from build123d import *

# Parameters (mm, degrees)
SKETCH1_W           = 25.4
SKETCH1_H           = 88.9
BOSS_EXTRUDE1_DEPTH = 30.226
SKETCH2_R           = 3.175
CUT_EXTRUDE1_DEPTH  = 12.7
SKETCH3_R           = 8.763
CUT_EXTRUDE2_DEPTH  = 3.556
CUT_EXTRUDE3_START  = -21.844
SKETCH4_R           = 10.795
CUT_EXTRUDE3_DEPTH  = 21.844
SKETCH5_W           = 54.61
SKETCH5_H           = 30.226
BOSS_EXTRUDE2_DEPTH = 3.175
SKETCH6_R           = 1.5875
CUT_EXTRUDE4_DEPTH  = 3.175
BOSS_EXTRUDE3_START = 2.54
SKETCH8_R           = 10.795
SKETCH8_R_2         = 6.35
BOSS_EXTRUDE3_DEPTH = 2.54
BOSS_EXTRUDE4_START = 19.304
SKETCH9_R           = 10.795
BOSS_EXTRUDE4_DEPTH = 19.304
SKETCH10_R          = 8.763
BOSS_EXTRUDE5_DEPTH = 10.16
SKETCH12_R          = 4.445
CUT_EXTRUDE5_DEPTH  = 12.7


with BuildPart() as part:
    # Sketch1 → Boss-Extrude1 (new body)
    with BuildSketch(Plane.XY):
        Rectangle(SKETCH1_W, SKETCH1_H)
    extrude(amount=BOSS_EXTRUDE1_DEPTH)

    # Sketch2 → Cut-Extrude1 (cut)
    with BuildSketch(Plane(origin=(12.7, 0, 0), x_dir=(0, 0, -1), z_dir=(1, 0, 0))):
        with Locations((-15.113, 38.1)):
            Circle(SKETCH2_R)
        with Locations((-15.113, -38.1)):
            Circle(SKETCH2_R)
    extrude(amount=-CUT_EXTRUDE1_DEPTH, mode=Mode.SUBTRACT)

    # Sketch3 → Cut-Extrude2 (cut)
    with BuildSketch(Plane(origin=(12.7, 0, 0), x_dir=(0, 0, -1), z_dir=(1, 0, 0))):
        with Locations((-15.113, 0)):
            Circle(SKETCH3_R)
    extrude(amount=-CUT_EXTRUDE2_DEPTH, mode=Mode.SUBTRACT)

    # Sketch4 → Cut-Extrude3 (cut)
    with BuildSketch(Plane(origin=(9.144, 0, 0), x_dir=(0, 0, -1), z_dir=(1, 0, 0)).offset(CUT_EXTRUDE3_START)):
        with Locations((-15.113, 0)):
            Circle(SKETCH4_R)
    extrude(amount=CUT_EXTRUDE3_DEPTH, mode=Mode.SUBTRACT)

    # Sketch5 → Boss-Extrude2 (add)
    with BuildSketch(Plane.XZ.offset(44.45)):
        with Locations((0, 15.113)):
            Rectangle(SKETCH5_W, SKETCH5_H)
    extrude(amount=BOSS_EXTRUDE2_DEPTH)

    # Sketch6 → Cut-Extrude4 (cut)
    with BuildSketch(Plane.XZ.offset(47.625)):
        with Locations(Location((-23.495, 25.908, 0), (0, 0, 270))):
            Circle(SKETCH6_R)
        with Locations(Location((-23.495, 4.318, 0), (0, 0, 270))):
            Circle(SKETCH6_R)
        with Locations(Location((23.495, 4.318, 0), (0, 0, 270))):
            Circle(SKETCH6_R)
        with Locations(Location((23.495, 25.908, 0), (0, 0, 270))):
            Circle(SKETCH6_R)
    extrude(amount=-CUT_EXTRUDE4_DEPTH, mode=Mode.SUBTRACT)

    # Sketch8 → Boss-Extrude3 (add)
    with BuildSketch(Plane.ZY.offset(-9.144).offset(BOSS_EXTRUDE3_START)):
        with Locations(Location((15.113, 0, 0), (0, 0, 180))):
            Circle(SKETCH8_R)
        with Locations((15.113, 0)):
            Circle(SKETCH8_R_2, mode=Mode.SUBTRACT)
    extrude(amount=-BOSS_EXTRUDE3_DEPTH)

    # Sketch9 → Boss-Extrude4 (add)
    with BuildSketch(Plane.ZY.offset(-6.604).offset(BOSS_EXTRUDE4_START)):
        with Locations((15.113, 0)):
            Circle(SKETCH9_R)
    extrude(amount=-BOSS_EXTRUDE4_DEPTH)

    # Sketch10 → Boss-Extrude5 (add)
    with BuildSketch(Plane(origin=(9.144, 0, 0), x_dir=(0, 0, -1), z_dir=(1, 0, 0))):
        with Locations((-15.113, 0)):
            Circle(SKETCH10_R)
    extrude(amount=-BOSS_EXTRUDE5_DEPTH)

    # Sketch12 → Cut-Extrude5 (cut)
    with BuildSketch(Plane(origin=(12.7, 0, 0), x_dir=(0, 0, -1), z_dir=(1, 0, 0))):
        with Locations((-15.113, 0)):
            Circle(SKETCH12_R)
    extrude(amount=-CUT_EXTRUDE5_DEPTH, mode=Mode.SUBTRACT)


solid = part.part
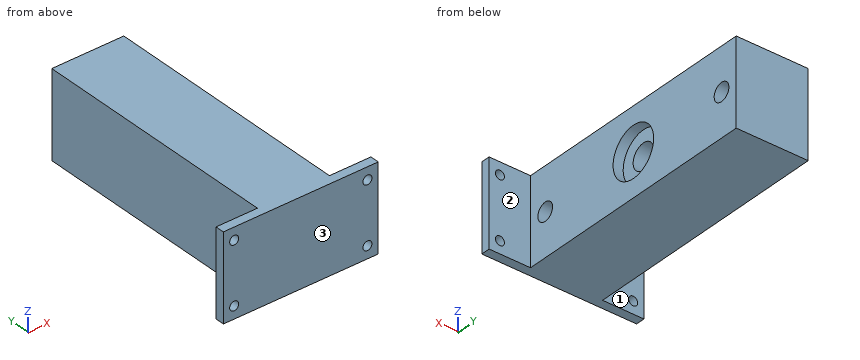
For this review, take the finished solid that the model builds, in its own axes (mm). Face numbers are marked on the shaded views. A direction names the side the tool comes from. Round coordinates to 2 decimals unless told otherwise and drop trailing zeros. Loops run counter-clockwise (first coordinate to the right, second up) from the corner with the lowest first, then second, coordinate; pieces in that order, holes last. Notation, with made-up numbers: (63.5, 66) - (120.5, 66) arc R31 ccw to (120.5, 101) - close; hole circle Ø11 at (35, 2). An arc over 180 degrees is marked (long way). One line per item, written item: value. Start each with the question number.
Item 1: For L1, parallel to Z at x = 4, y = -38; L2, parallel to X at y = -22.5, z = 9; L3, parallel to Y at x = -16, z = 12.5 (3 decimals), list the stretches that pass through material, from the lowest coordinate up.
Item 2: Take a section at B-B (x = 7). Give the boundary of the cut face in (y, z) (3 decimals).
Item 3: Take a section at A-A (y = 0). Give the boundary of the cut face in (x, z), plus the area to 3 significant figures.
Item 4: Take a section at C-C (z = 26). Give the boundary of the cut face in (x, y) (3 decimals).
Item 5: Clearance check with flat-ended pins moving along their axes: pin 1 Ø4 at (x, y) = (-12.5, 11) entering from -Z; pin 2 Ø9 at (y, z) = (19.5, 16) entering from -X; pin 3 Ø2 at (y, z) = (9, 8.5) entering from +X; pin 4 Ø11.5 at (x, z) = (21, 14.5) entering from +Y. State where each tip first meets the part, or that it passes through.
Item 6: Take a section at D-D (y = -38.1). Give the boundary of the cut face in (x, z), plus the area to 3 significant figures.
Item 7: For the marked faces 1, 2 and 3, list the 3-axis set-ups (+Z, -Z, +X, -X, +Y, -Y) from which the entire face can be reached by the end or side of a thin tool; tool diameter is ignored.
Answer below:
1. L1: z = 0 to 11.94, 18.29 to 30.23
1. L2: x = -12.7 to 12.7
1. L3: y = -47.625 to -44.45
2. outline: (-47.625, 0) - (44.45, 0) - (44.45, 30.226) - (-47.625, 30.226) - close; hole circle Ø6.35 at (-38.1, 15.113); hole circle Ø8.89 at (0, 15.113); hole circle Ø6.35 at (38.1, 15.113)
3. outline: (-12.7, 0) - (12.7, 0) - (12.7, 6.35) - (9.14, 6.35) - (9.14, 10.67) - (0, 10.67) - (0, 19.56) - (9.14, 19.56) - (9.14, 23.88) - (12.7, 23.88) - (12.7, 30.23) - (-12.7, 30.23) - close
3. area: 624 mm2
4. outline: (-27.305, -47.625) - (-25.08, -47.625) - (-25.08, -44.45) - (-27.305, -44.45) - close; (-21.91, -47.625) - (21.91, -47.625) - (21.91, -44.45) - (12.7, -44.45) - (12.7, 44.45) - (-12.7, 44.45) - (-12.7, -44.45) - (-21.91, -44.45) - close; (25.08, -47.625) - (27.305, -47.625) - (27.305, -44.45) - (25.08, -44.45) - close
5. pin 1: stops at z = 0
5. pin 2: stops at x = -12.7
5. pin 3: stops at x = 12.7
5. pin 4: stops at y = -44.45
6. outline: (-12.7, 0) - (12.7, 0) - (12.7, 11.94) - (0, 11.94) - (0, 18.29) - (12.7, 18.29) - (12.7, 30.23) - (-12.7, 30.23) - close
6. area: 687 mm2
7. face 1: +Z, -Z, -X, +Y
7. face 2: +Z, -Z, +X, +Y
7. face 3: +Z, -Z, +X, -X, -Y
